For this review, take the finished solid that the model builds, in its own axes (mm). Round coordinates to 2 decimals unless told otherwise and drop trailing zeros. Loops run counter-clockwise (first coordinate to the right, second up) from the corner with the lowest first, then second, coordinate; pieces in that order, holes last.
1. Consider section C-C on x = 0. State the section outline as (y, z) points.
2. Consider section B-B on y = -25. State the section outline as (x, z) points, then the cut area to 3 significant figures.
3. To check wall thickness, follow line 1 along Y through (x, z) = (0, 3); line 2 along Z through (x, y) = (31, -15.5); line 3 along Y through (x, z) = (-0.5, 13.5). State the ranges of each line that lie inside material, in increasing order.
4. Clearance check with flat-ended pins moving along their axes: pin 1 Ø4 at (x, z) = (-33, 17.5) entering from -Y; pin 2 Ø23 at (x, z) = (-60, 22) entering from +Y; pin 3 Ø9.5 at (x, y) = (50, 0) entering from -Z; pin 4 Ø15.5 at (x, y) = (0, 25) entering from +Z. State where each tip first meets the part, or that it passes through.
5. Consider section A-A on y = 0. State the section outline as (x, z) points, then the cut area to 3 significant figures.
6. Consider section D-D on z = 22. State the section outline as (x, y) points, then the cut area to 3 significant figures.
7. Draft analysis for pull direction X (two halves, no side actions). For faces 1 (the flat face through (-17.912, -16, 5)), 2 (the cylindrical face through (-6.56, 41.76, 4.93)), 3 (the cylindrical face through (44, 0, 5)), state which applies: released by +X, released by -X, zero draft, split by the parting line, or undercut.
from build123d import *

# Parameters (mm, degrees)
F0_R          = 6
F1_DEPTH      = 10
F2_R          = 10
F3_DEPTH      = 8
F3_DEPTH_BACK = 8


with BuildPart() as f1:
    # F0 (on Top) → F1 (new body)
    with BuildSketch(Plane.XY):
        with BuildLine():
            ThreePointArc((50.720724, 17.985565), (30.362055, 23.224109), (13.956018, 36.367918))
            ThreePointArc((13.956018, 36.367918), (-6.862265, 41.640593), (-17.912368, 23.226))
            Line((-17.912368, 23.226), (-17.912368, -23.226))
            ThreePointArc((-17.912368, -23.226), (-6.862265, -41.640593), (13.956018, -36.367918))
            ThreePointArc((13.956018, -36.367918), (30.362055, -23.224109), (50.720724, -17.985565))
            ThreePointArc((50.720724, -17.985565), (68, 0), (50.720724, 17.985565))
        make_face()
        with Locations((0, -25)):
            Circle(F0_R, mode=Mode.SUBTRACT)
        with Locations((0, 25)):
            Circle(F0_R, mode=Mode.SUBTRACT)
        with Locations((50, 0)):
            Circle(F0_R, mode=Mode.SUBTRACT)
    extrude(amount=F1_DEPTH)

    # F2 (on Front) → F3 (join, two sides)
    with BuildSketch(Plane.XZ) as f3_sk:
        with BuildLine():
            ThreePointArc((24.938122, 10), (-12.836551, 20.714776), (-47.128021, 39.841393))
            ThreePointArc((-47.128021, 39.841393), (-80.934426, 28.763481), (-59.999878, 0))
            Line((-59.999878, 0), (24.938122, 0))
            Line((24.938122, 0), (24.938122, 10))
        make_face()
        with Locations((-59.999878, 22)):
            Circle(F2_R, mode=Mode.SUBTRACT)
    extrude(amount=F3_DEPTH)
    extrude(f3_sk.sketch, amount=-F3_DEPTH_BACK)


solid = f1.part
Resolved:
1. outline: (-43, 0) - (-31, 0) - (-31, 10) - (-43, 10) - close; (-19, 0) - (19, 0) - (19, 10) - (8, 10) - (8, 16) - (-8, 16) - (-8, 10) - (-19, 10) - close; (31, 0) - (43, 0) - (43, 10) - (31, 10) - close
2. outline: (-18, 0) - (-6, 0) - (-6, 10) - (-18, 10) - close; (6, 0) - (27.12, 0) - (27.12, 10) - (6, 10) - close
2. area: 331 mm2
3. line 1: y = -43 to -31, -19 to 19, 31 to 43
3. line 2: z = 0 to 10
3. line 3: y = -8 to 8
4. pin 1: stops at y = -8
4. pin 2: stops at y = 8
4. pin 3: passes through
4. pin 4: stops at z = 10
5. outline: (-60, 0) - (44, 0) - (44, 10) - (24.94, 10) arc R169.34 cw to (-47.13, 39.84) arc R22 ccw (long way) to start; (56, 0) - (68, 0) - (68, 10) - (56, 10) - close; hole circle Ø20 at (-60, 22)
5. area: 2,860 mm2
6. outline: (-82, -8) - (-70, -8) - (-70, 8) - (-82, 8) - close; (-50, -8) - (-15.86, -8) - (-15.86, 8) - (-50, 8) - close
6. area: 738 mm2
7. face 1: released by -X
7. face 2: split by the parting line
7. face 3: undercut
